Job drawing, mm, ordinate dimensions from the low corner. One solid piece. Coordinates: 2 decimals unless noted, no trailing zeros. Write each loop counter-clockwise with the first axis right and the second up, starting at its lowest first coordinate (ties: lowest second). Pieces come first, ordered by that corner, then holes.
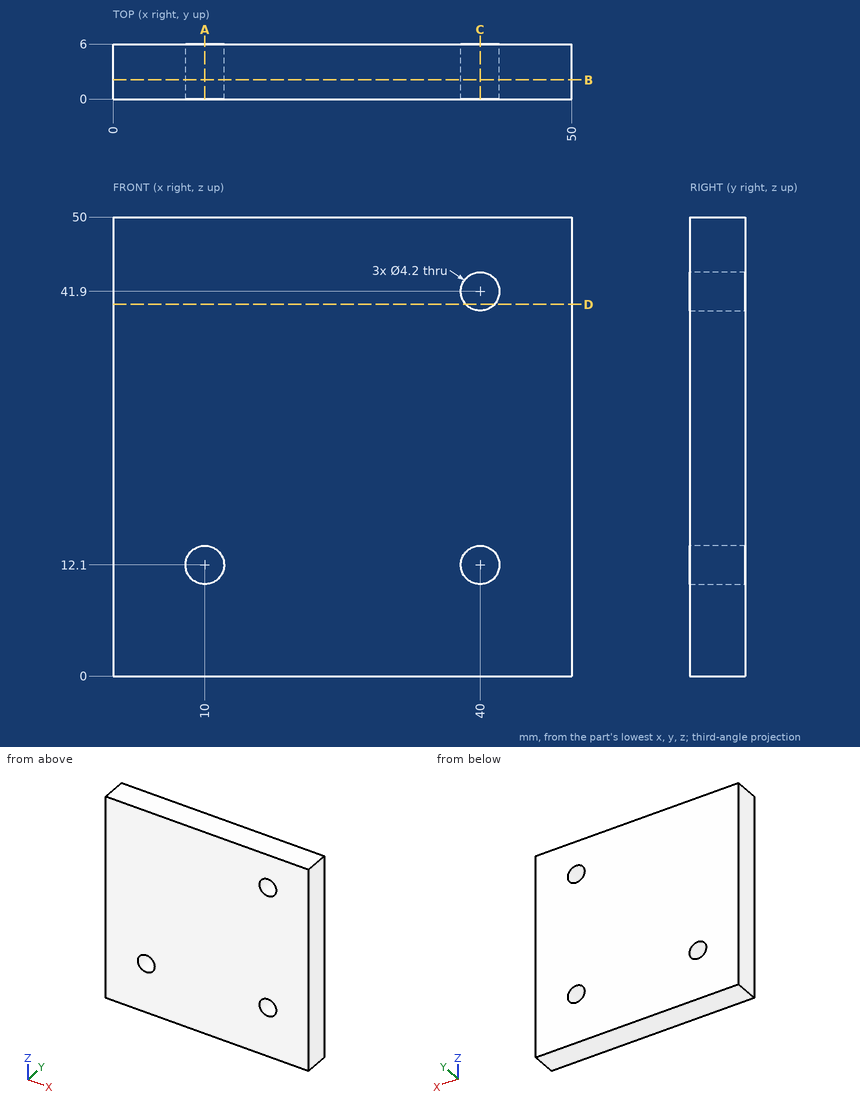
1. Saw through at D-D on z = 40.5. List the corners of the cut face in (x, y), plus the area to 3 significant figures.
Computed values:
outline: (0, 0) - (38.43, 0) - (38.43, 6) - (0, 6) - close; (41.57, 0) - (50, 0) - (50, 6) - (41.57, 6) - close
area: 281 mm2
2. Saw through at B-B on y = 2.1. List the corners of the cut face in (x, z).
Computed values:
outline: (0, 0) - (50, 0) - (50, 50) - (0, 50) - close; hole circle Ø4.2 at (10, 12.1); hole circle Ø4.2 at (40, 12.1); hole circle Ø4.2 at (40, 41.9)
3. Saw through at A-A on x = 10. List the corners of the cut face in (y, z), plus the area to 3 significant figures.
Computed values:
outline: (0, 0) - (6, 0) - (6, 10) - (0, 10) - close; (0, 14.2) - (6, 14.2) - (6, 50) - (0, 50) - close
area: 275 mm2
4. Probe line 1 along X through (y, z) = (3.05, 12.1). List the from-to ranges inside material, lowest first.
Computed values:
line 1: x = 0 to 7.9, 12.1 to 37.9, 42.1 to 50
5. Saw through at C-C on x = 40. List the corners of the cut face in (y, z).
Computed values:
outline: (0, 0) - (6, 0) - (6, 10) - (0, 10) - close; (0, 14.2) - (6, 14.2) - (6, 39.8) - (0, 39.8) - close; (0, 44) - (6, 44) - (6, 50) - (0, 50) - close
